```python
from build123d import *

# Parameters (mm, degrees)
MODEL_R                  = 2.1
MODEL_R_2                = 3.4
STRUCTURAL_MEMBER1_DEPTH = 36


with BuildPart() as part:
    # Model → Structural Member1 (new body)
    with BuildSketch(Plane(origin=(0, 0, 0), x_dir=(-1, 0, 0), z_dir=(0, 1, 0))):
        with BuildLine():
            Line((-15, 13), (-15, 4.3))
            ThreePointArc((-15, 4.3), (-14.912132034, 4.087867966), (-14.7, 4))
            Line((-14.7, 4), (-13, 4))
            Line((-13, 4), (-13, 8.25))
            Line((-13, 8.25), (-9.6642, 8.25))
            Line((-9.6642, 8.25), (-6, 4.5858))
            Line((-6, 4.5858), (-6, 0.519615242))
            Line((-6, 0.519615242), (-5.7, 0))
            Line((-5.7, 0), (-6, -0.519615242))
            Line((-6, -0.519615242), (-6, -4.5858))
            Line((-6, -4.5858), (-9.6642, -8.25))
            Line((-9.6642, -8.25), (-13, -8.25))
            Line((-13, -8.25), (-13, -4))
            Line((-13, -4), (-14.7, -4))
            ThreePointArc((-14.7, -4), (-14.912132034, -4.087867966), (-15, -4.3))
            Line((-15, -4.3), (-15, -13))
            ThreePointArc((-15, -13), (-14.414213562, -14.414213562), (-13, -15))
            Line((-13, -15), (-4.3, -15))
            ThreePointArc((-4.3, -15), (-4.087867966, -14.912132034), (-4, -14.7))
            Line((-4, -14.7), (-4, -13))
            Line((-4, -13), (-8.25, -13))
            Line((-8.25, -13), (-8.25, -9.6642))
            Line((-8.25, -9.6642), (-4.5858, -6))
            Line((-4.5858, -6), (-0.519615242, -6))
            Line((-0.519615242, -6), (0, -5.7))
            Line((0, -5.7), (0.519615242, -6))
            Line((0.519615242, -6), (4.5858, -6))
            Line((4.5858, -6), (8.25, -9.6642))
            Line((8.25, -9.6642), (8.25, -13))
            Line((8.25, -13), (4, -13))
            Line((4, -13), (4, -14.7))
            ThreePointArc((4, -14.7), (4.087867966, -14.912132034), (4.3, -15))
            Line((4.3, -15), (13, -15))
            ThreePointArc((13, -15), (14.414213562, -14.414213562), (15, -13))
            Line((15, -13), (15, -4.3))
            ThreePointArc((15, -4.3), (14.912132034, -4.087867966), (14.7, -4))
            Line((14.7, -4), (13, -4))
            Line((13, -4), (13, -8.25))
            Line((13, -8.25), (9.6642, -8.25))
            Line((9.6642, -8.25), (6, -4.5858))
            Line((6, -4.5858), (6, -0.519615242))
            Line((6, -0.519615242), (5.7, 0))
            Line((5.7, 0), (6, 0.519615242))
            Line((6, 0.519615242), (6, 4.5858))
            Line((6, 4.5858), (9.6642, 8.25))
            Line((9.6642, 8.25), (13, 8.25))
            Line((13, 8.25), (13, 4))
            Line((13, 4), (14.7, 4))
            ThreePointArc((14.7, 4), (14.912132034, 4.087867966), (15, 4.3))
            Line((15, 4.3), (15, 13))
            ThreePointArc((15, 13), (14.414213562, 14.414213562), (13, 15))
            Line((13, 15), (4.3, 15))
            ThreePointArc((4.3, 15), (4.087867966, 14.912132034), (4, 14.7))
            Line((4, 14.7), (4, 13))
            Line((4, 13), (8.25, 13))
            Line((8.25, 13), (8.25, 9.6642))
            Line((8.25, 9.6642), (4.5858, 6))
            Line((4.5858, 6), (0.519615242, 6))
            Line((0.519615242, 6), (0, 5.7))
            Line((0, 5.7), (-0.519615242, 6))
            Line((-0.519615242, 6), (-4.5858, 6))
            Line((-4.5858, 6), (-8.25, 9.6642))
            Line((-8.25, 9.6642), (-8.25, 13))
            Line((-8.25, 13), (-4, 13))
            Line((-4, 13), (-4, 14.7))
            ThreePointArc((-4, 14.7), (-4.087867966, 14.912132034), (-4.3, 15))
            Line((-4.3, 15), (-13, 15))
            ThreePointArc((-13, 15), (-14.414213562, 14.414213562), (-15, 13))
        make_face()
        with Locations((11.625, -11.625)):
            Circle(MODEL_R, mode=Mode.SUBTRACT)
        with Locations((11.625, 11.625)):
            Circle(MODEL_R, mode=Mode.SUBTRACT)
        Circle(MODEL_R_2, mode=Mode.SUBTRACT)
        with Locations((-11.625, -11.625)):
            Circle(MODEL_R, mode=Mode.SUBTRACT)
        with Locations((-11.625, 11.625)):
            Circle(MODEL_R, mode=Mode.SUBTRACT)
    extrude(amount=STRUCTURAL_MEMBER1_DEPTH)


solid = part.part
```
Work out the finished part from the listing and answer in its coordinate system (mm). A direction names the side the tool comes from. Give positions to 0.01 mm unless a question says otherwise; leave off trailing zeros. Loops run counter-clockwise (first coordinate to the right, second up) from the corner with the lowest first, then second, coordinate; pieces in that order, holes last. Notation, with made-up numbers: (62, -26.75) -> (94, -26.75) arc R33 ccw to (94, 2.25) -> close; hole circle Ø5 at (38.25, -7). An arc over 180 degrees is marked (long way). Write item = value, one per line. Start each with the question number.
(1) Find the intervals of material crossed by probe 1 along X at (y, z) = (22, -4.5); probe 2 along Z at (x, y) = (5.75, 8.5), in increasing order. Write a range as from..to.
(2) Find section B-B on z = -7.5. Give the vertices of the cut face in (x, y), and give its area (3 significant figures).
(3) The mould has two halves that part along X. Classify faces 5 (the flat face through (-3, 18, -6)), 6 (the flat face through (15, 18, -9)), 7 (the flat face through (14, 18, 4)): +X half, -X half, draft (parallel to the pull), parting line (faces both ways), or undercut.
(4) Find section D-D on y = 13.5. Give the number of separate pieces and of enclosed holes in the cut face, and give its area (3 significant figures).
(5) Find section A-A on z = 1.5. Give the vertices of the cut face in (x, y), and give its area (3 significant figures).
(6) Find section C-C on z = 10.5. Give the vertices of the cut face in (x, y), and give its area (3 significant figures).
(7) Given pin 1 Ø4.5 at (y, z) = (23.5, -2) entering from +X; pin 2 Ø0.8 at (y, z) = (24, -14) entering from -X; pin 3 Ø0.8 at (y, z) = (18, 14) entering from +X; pin 4 Ø2.5 at (x, z) = (11.625, 11.625) entering from -Y (3 decimals), each flat-ended and moving along its own axis, determine where each tip first touches the part or whether it passes through.
(8) Which of the six approach directions +Z, -Z, +X, -X, +Y, -Y give full straight-line access (tool end or side, diameter ignored) to faces 1 (the cylindrical face through (14.43, 17.75, -14.4)), 2 (the flat face through (-11, 18, 8.25)), 3 (the flat face through (-4, 18, 14)), 4 (the flat face through (14, 18, -4))?
From the geometry:
q1.probe_1 = -15..-13, -6..6, 13..15
q1.probe_2 = -15..-13, -7.16..-0.09, 0.09..7.16, 13..15
q2.outline = (-15, 0) -> (-13, 0) -> (-13, 36) -> (-15, 36) -> close; (-8.91, 0) -> (-6.09, 0) -> (-6.09, 36) -> (-8.91, 36) -> close; (6.09, 0) -> (8.91, 0) -> (8.91, 36) -> (6.09, 36) -> close; (13, 0) -> (15, 0) -> (15, 36) -> (13, 36) -> close
q2.area = 348 mm^2
q3.face_5 = undercut
q3.face_6 = +X half
q3.face_7 = draft
q4.separate_pieces = 1
q4.enclosed_holes = 5
q4.area = 332 mm^2
q5.outline = (-6, 0) -> (-3.05, 0) -> (-3.05, 36) -> (-6, 36) -> close; (3.05, 0) -> (6, 0) -> (6, 36) -> (3.05, 36) -> close
q5.area = 212 mm^2
q6.outline = (-15, 0) -> (-13.4, 0) -> (-13.4, 36) -> (-15, 36) -> close; (-9.85, 0) -> (-8.25, 0) -> (-8.25, 36) -> (-9.85, 36) -> close; (8.25, 0) -> (9.85, 0) -> (9.85, 36) -> (8.25, 36) -> close; (13.4, 0) -> (15, 0) -> (15, 36) -> (13.4, 36) -> close
q6.area = 231 mm^2
q7.pin_1 = 15
q7.pin_2 = -14.91
q7.pin_3 = 14.91
q7.pin_4 = through
q8.face_1 = -Z, +X, +Y, -Y
q8.face_2 = +Y, -Y
q8.face_3 = +Z, +Y, -Y
q8.face_4 = +X, +Y, -Y
